CAD build for the part. Positions are in the model's coordinates, mm. Face numbers are marked on the shaded views. A direction names the side the tool comes from. Coordinates: 2 decimals unless noted, no trailing zeros. Write each loop counter-clockwise with the first axis right and the second up, starting at its lowest first coordinate (ties: lowest second). Pieces come first, ordered by that corner, then holes. Notation, with made-up numbers: (18.5, 61.5) - (61.5, 61.5) arc R15 ccw to (61.5, 80.5) - close; hole circle Ø8 at (34, -12). An arc over 180 degrees is marked (long way). One line per question, with ' | ' between items. Start each with the question number.
1. Band-saw the part on D-D, the plane x = -3.5. Write the cut outline in (y, z), then the cut area to 3 significant figures.
2. Flat gauge pin, fed straight in: P1, Ø2, axis at x = 0.5, z = 1, coming from the +Y side. Where does the tip first touch, or does it go through?
3. Band-saw the part on A-A, the plane y = -4. Write the cut outline in (x, z), then the cut area to 3 significant figures.
4. Which spindle directions (+Z, -Z, +X, -X, +Y, -Y) get a long thin tool onto all of the face, cutting with end or side? Do the marked faces 4 and 5. Say none if no direction does.
5. Band-saw the part on B-B, the plane x = 0. Write the cut outline in (y, z).
6. Band-saw the part on C-C, the plane z = 2.6. Write the cut outline in (x, y), then the cut area to 3 significant figures.
7. Probe line 1 (Y direction, x = 0, z = 2.6); line 2 (X direction, y = 9.5, z = 2.45); line 3 (Y direction, x = -0.5, z = 2.9). List the from-to ranges inside material, lowest first.
8. Two-plate mould, pull along Y, no slides. Class the marked faces 1, 2 and 3: +Y half, -Y half, draft (parallel to the pull), parting line (faces both ways), or undercut.
Autodesk Inventor part; units mm, degrees
ref_plane "YZ Plane" through (0, 0, 0) normal (1, 0, 0) x (0, 1, 0)
ref_plane "XZ Plane" through (0, 0, 0) normal (0, 1, 0) x (-1, 0, 0)
ref_plane "XY Plane" through (0, 0, 0) normal (0, 0, 1) x (1, 0, 0)
sketch "Sketch1" plane through (0, 0, 0) normal (0, 0, 1) x (1, 0, 0)
  line L0 (0, 15) -> (0, -15) construction
  line L1 (-4, 15) -> (-4, -15)
  line L2 (4, -15) -> (4, 15)
  arc A0 (4, 15) -> (-4, 15) centre (0, 15) ccw
  arc A1 (-4, -15) -> (4, -15) centre (0, -15) ccw
  circle A2 centre (0, -15) radius 1.5
  line L3 (0, -5) -> (0, 15) construction
  line L4 (1.5, -5) -> (1.5, 15)
  line L5 (-1.5, 15) -> (-1.5, -5)
  arc A3 (-1.5, -5) -> (1.5, -5) centre (0, -5) ccw
  arc A4 (1.5, 15) -> (-1.5, 15) centre (0, 15) ccw
  point P0 (0, 0)
  point P1 (0, 5)
  dimension "d0" = 15
  dimension "d1" = 8
  dimension "d2" = 3
  dimension "d3" = 10
  dimension "d4" = 3
  dimension "d5" = 10
extrude "Extrusion1" add sketch "Sketch1" along normal blind 3.5
properties part number "3DP_PLA_Measurement_Rail_Mounting_Bracket_Short" material "ABS Plastic"
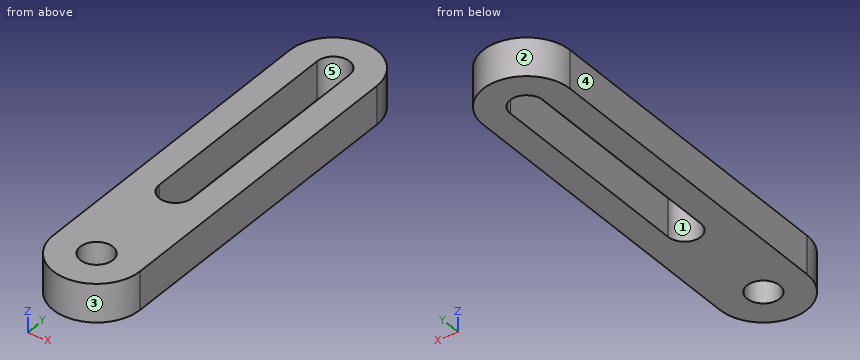
Filled in:
1) outline: (-16.94, 0) - (16.94, 0) - (16.94, 3.5) - (-16.94, 3.5) - close | area: 119 mm²
2) P1: stops at y = 19
3) outline: (-4, 0) - (-1.5, 0) - (-1.5, 3.5) - (-4, 3.5) - close; (1.5, 0) - (4, 0) - (4, 3.5) - (1.5, 3.5) - close | area: 17.5 mm²
4) face 4: +Z, -Z, -X, +Y, -Y | face 5: +Z, -Z
5) outline: (-19, 0) - (-16.5, 0) - (-16.5, 3.5) - (-19, 3.5) - close; (-13.5, 0) - (-6.5, 0) - (-6.5, 3.5) - (-13.5, 3.5) - close; (16.5, 0) - (19, 0) - (19, 3.5) - (16.5, 3.5) - close
6) outline: (-4, -15) arc R4 ccw to (4, -15) - (4, 15) arc R4 ccw to (-4, 15) - close; hole circle Ø3 at (0, -15); hole (-1.5, -5) arc R1.5 ccw to (1.5, -5) - (1.5, 15) arc R1.5 ccw to (-1.5, 15) - close | area: 216 mm²
7) line 1: y = -19 to -16.5, -13.5 to -6.5, 16.5 to 19 | line 2: x = -4 to -1.5, 1.5 to 4 | line 3: y = -18.97 to -16.41, -13.59 to -6.41, 16.41 to 18.97
8) face 1: undercut | face 2: +Y half | face 3: -Y half
